Work out the finished part from the listing and answer in its coordinate system (mm). A direction names the side the tool comes from. Round coordinates to 2 decimals unless told otherwise and drop trailing zeros. Write each loop counter-clockwise with the first axis right and the second up, starting at its lowest first coordinate (ties: lowest second). Pieces come first, ordered by that corner, then holes. Notation, with made-up numbers: M -9.5,19 L 37.5,19 A33 ccw 37.5,47 Z; hole C -9.5,65.25 d1. An arc over 180 degrees is marked long. One line per item, written item: value. Start each with the question number.
Q1. Consider probe 1 along Z at (x, y) = (-2, -7.5); probe 2 along Y at (x, z) = (-15.5, 4); probe 3 along X at (y, z) = (-7, 13). Determine where each line is inside the solid, lowest interval first.
Q2. Find section D-D (x = -19). Write down the section's boundary in (y, z).
Q3. Given pin 1 Ø2 at (y, z) = (-9.5, 18.5) entering from -X; pin 2 Ø5 at (x, z) = (-18, 13.5) entering from +Y, each flat-ended and moving along its own axis, determine where each tip first touches the part or whether it passes through.
Q4. Find section A-A (z = 6). Write down the section's boundary in (x, y), and give its area (3 significant figures).
Q5. A tool of negligible diameter and unlimited length cuts with its end or side. For faces 1 (the flat face through (-7.5, -12, 10)), 2 (the flat face through (-24.5, -26, 10)), from which of +Z, -Z, +X, -X, +Y, -Y can it reach the whole face along a straight path? Write none if from no direction.
Q6. Find section B-B (x = 0). Write down the section's boundary in (y, z).
Q7. Find section C-C (y = -21). Write down the section's boundary in (x, z).
from build123d import *
from build123d.topology import SkipClean

# Parameters (mm, degrees)
BOSS_EXTRUDE1_DEPTH = 20
SKETCH3_R           = 7.5
BOSS_EXTRUDE3_DEPTH = 8


with BuildPart() as part:
    # Sketch1 → Boss-Extrude1 (new body)
    with BuildSketch(Plane.XY):
        with BuildLine():
            Line((7.5, 0), (7.5, -29))
            Line((7.5, -29), (-24.5, -29))
            Line((-24.5, -29), (-24.5, -23))
            Line((-24.5, -23), (-7.5, -23))
            Line((-7.5, -23), (-7.5, 0))
            ThreePointArc((-7.5, 0), (0, 7.5), (7.5, 0))
        make_face()
    extrude(amount=BOSS_EXTRUDE1_DEPTH)

    # Sketch3 → Boss-Extrude3 (add)
    with SkipClean():  # the faces are left unmerged after this step: merging them gives an invalid solid
        with BuildSketch(Plane.XY.offset(20)):
            Circle(SKETCH3_R)
        extrude(amount=BOSS_EXTRUDE3_DEPTH)
    add(part.part.scale(1), mode=Mode.REPLACE)  # the faces are merged on a copy


solid = part.part
The answers:
1. probe 1: 0 to 20
1. probe 2: -29 to -23
1. probe 3: -7.5 to 7.5
2. outline: M -29,0 L -23,0 L -23,20 L -29,20 Z
3. pin 1: x = -7.5
3. pin 2: y = -23
4. outline: M -24.5,-29 L 7.5,-29 L 7.5,0 A7.5 ccw -7.5,0 L -7.5,-23 L -24.5,-23 Z
4. area: 625 mm2
5. face 1: +Z, -Z, -X, +Y
5. face 2: +Z, -Z, -X, +Y, -Y
6. outline: M -29,0 L 7.5,0 L 7.5,28 L -7.5,28 L -7.5,20 L -29,20 Z
7. outline: M -7.5,0 L 7.5,0 L 7.5,20 L -7.5,20 Z
